Geometry check sheet. Reference: the model listing, model coordinates, mm. Face numbers are marked on the shaded views. A direction names the side the tool comes from. Coordinates: 2 decimals unless noted, no trailing zeros. Order: outer loops, then holes, each group sorted by start corner. A loop starts at its lowest first (then second) coordinate and runs counter-clockwise, first axis right, second up. Notation, with made-up numbers: (77.25, 26.25) - (81.25, 26.25) arc R29 cw to (81.25, 65.25) - close; hole circle Ø3 at (-25, 85.5). An arc over 180 degrees is marked (long way). One line per item, written item: value. Start each with the question number.
```python
from build123d import *

# Parameters (mm, degrees)
SKETCH1_R           = 18.1
SKETCH1_R_2         = 1.55
SKETCH1_R_3         = 6.05
BOSS_EXTRUDE1_DEPTH = 1
SKETCH2_W           = 38.2
SKETCH2_H           = 38.2
SKETCH2_R           = 18.1
BOSS_EXTRUDE2_DEPTH = 46
SKETCH3_W           = 10
SKETCH3_H           = 15
SKETCH3_R           = 1.55
BOSS_EXTRUDE3_DEPTH = 2


with BuildPart() as part:
    # Sketch1 → Boss-Extrude1 (new body)
    with BuildSketch(Plane.XY):
        Circle(SKETCH1_R)
        with Locations((15, 0)):
            Circle(SKETCH1_R_2, mode=Mode.SUBTRACT)
        with Locations((7.5, 12.990381057)):
            Circle(SKETCH1_R_2, mode=Mode.SUBTRACT)
        with Locations((-7.5, 12.990381057)):
            Circle(SKETCH1_R_2, mode=Mode.SUBTRACT)
        with Locations((0, 6)):
            Circle(SKETCH1_R_3, mode=Mode.SUBTRACT)
        with Locations((-15, 0)):
            Circle(SKETCH1_R_2, mode=Mode.SUBTRACT)
        with Locations((7.5, -12.990381057)):
            Circle(SKETCH1_R_2, mode=Mode.SUBTRACT)
        with Locations((-7.5, -12.990381057)):
            Circle(SKETCH1_R_2, mode=Mode.SUBTRACT)
    extrude(amount=BOSS_EXTRUDE1_DEPTH)

    # Sketch2 → Boss-Extrude2 (add)
    with BuildSketch(Plane(origin=(0, 0, 0), x_dir=(-1, 0, 0), z_dir=(0, 0, -1))):
        Rectangle(SKETCH2_W, SKETCH2_H)
        Circle(SKETCH2_R, mode=Mode.SUBTRACT)
    extrude(amount=-BOSS_EXTRUDE2_DEPTH)

    # Sketch3 → Boss-Extrude3 (add)
    with BuildSketch(Plane.XZ.offset(19.1)):
        with Locations((24.1, 7.5)):
            Rectangle(SKETCH3_W, SKETCH3_H)
        with Locations((24.5, 7.5)):
            Circle(SKETCH3_R, mode=Mode.SUBTRACT)
        with Locations((24.1, 38.5)):
            Rectangle(SKETCH3_W, SKETCH3_H)
        with Locations((24.5, 38.5)):
            Circle(SKETCH3_R, mode=Mode.SUBTRACT)
        with Locations((-24.1, 38.5)):
            Rectangle(SKETCH3_W, SKETCH3_H)
        with Locations((-24.5, 38.5)):
            Circle(SKETCH3_R, mode=Mode.SUBTRACT)
        with Locations((-24.1, 7.5)):
            Rectangle(SKETCH3_W, SKETCH3_H)
        with Locations((-24.5, 7.5)):
            Circle(SKETCH3_R, mode=Mode.SUBTRACT)
    boss_extrude3 = extrude(amount=-BOSS_EXTRUDE3_DEPTH)

    # Mirror1: Boss-Extrude3 across plane
    add(boss_extrude3.mirror(Plane.ZX))


solid = part.part
```
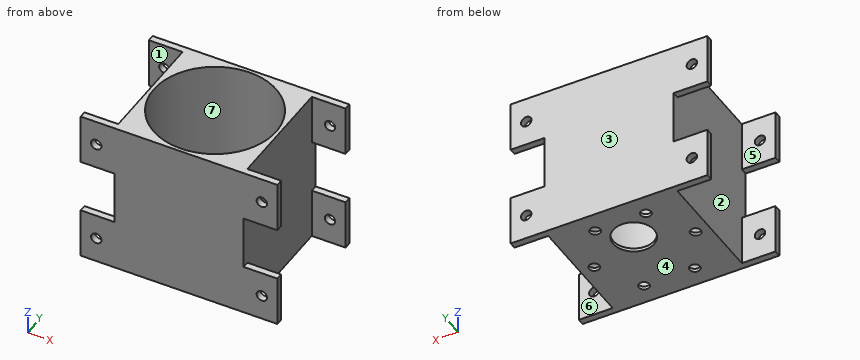
Q1. Set-up check for the marked faces 5, 6 and 7: record each of +Z, -Z, +X, -X, +Y, -Y from which the full face is reachable in a straight line by a thin tool's end or side.
Q2. Gauge pin test, flat ends, axial feed: P1, Ø5, axis at y = -13.5, z = 40, coming from the +X side; P2, Ø1, axis at y = -14.5, z = 11.5, coming from the -X side; P3, Ø3, axis at x = 3.5, y = 2.5, coming from the +Z side. Record the tip position at first contact, or that the pin passes through.
Q3. Cross-section at A-A, the plane z = 38.5. Count the separate pieces of the cut face and the enclosed holes in it, and give its area (3 significant figures).
Q4. Cross-section at B-B, the plane x = -20.5. Enter the section's corners in (y, z), and give its area (3 significant figures).
Q5. Material ranges on probe 1 along Z at (x, y) = (-24.5, -18); probe 2 along Y at (x, z) = (-7.5, 0.75); probe 3 along Y at (x, z) = (-3, 3), recorded low to high.
Q6. Release check for a two-part mould opening along Y. For the marked faces 1, 2, 3 and 4 record: released by +Y, released by -Y, zero draft, split by the parting line, or undercut.
Q7. Cross-section at D-D, the plane z = 11. Enter the section's corners in (x, y), and give its area (3 significant figures).
Check result:
1. face 5: +Z, -Z, -X
1. face 6: +Z, -Z, +X
1. face 7: +Z
2. P1: stops at x = 19.1
2. P2: stops at x = -19.1
2. P3: stops at z = 1
3. separate pieces: 5
3. enclosed holes: 1
3. area: 485 mm2
4. outline: (-19.1, 0) - (-17.1, 0) - (-17.1, 15) - (-19.1, 15) - close; (-19.1, 31) - (-17.1, 31) - (-17.1, 46) - (-19.1, 46) - close; (17.1, 0) - (19.1, 0) - (19.1, 15) - (17.1, 15) - close; (17.1, 31) - (19.1, 31) - (19.1, 46) - (17.1, 46) - close
4. area: 120 mm2
5. probe 1: z = 0 to 5.95, 9.05 to 15, 31 to 36.95, 40.05 to 46
5. probe 2: y = -19.1 to -14.54, -11.44 to 11.44, 14.54 to 19.1
5. probe 3: y = -19.1 to -17.85, 17.85 to 19.1
6. face 1: undercut
6. face 2: undercut
6. face 3: released by +Y
6. face 4: zero draft
7. outline: (-29.1, -19.1) - (29.1, -19.1) - (29.1, -17.1) - (19.1, -17.1) - (19.1, 17.1) - (29.1, 17.1) - (29.1, 19.1) - (-29.1, 19.1) - (-29.1, 17.1) - (-19.1, 17.1) - (-19.1, -17.1) - (-29.1, -17.1) - close; hole circle Ø36.2 at (0, 0)
7. area: 510 mm2
